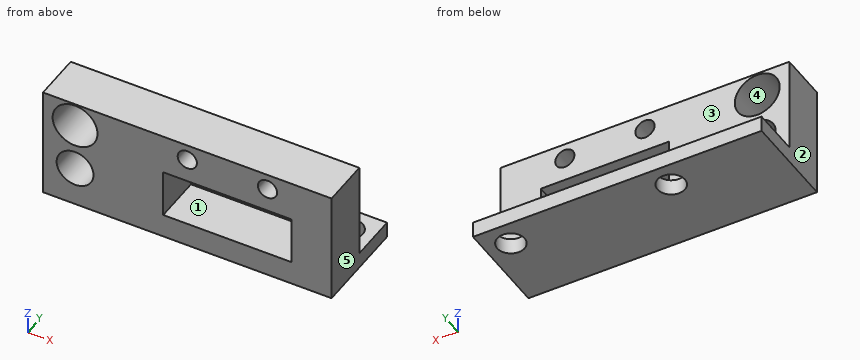
from build123d import *

# Parameters (mm, degrees)
SKETCH1_W           = 45.72
SKETCH1_H           = 17.78
BOSS_EXTRUDE1_DEPTH = 7.62
SKETCH2_W           = 45.72
SKETCH2_H           = 2.54
BOSS_EXTRUDE2_DEPTH = 7.62
SKETCH3_R           = 2.1717
CUT_EXTRUDE1_DEPTH  = 2.54
SKETCH4_R           = 3.556
SKETCH4_R_2         = 2.921
SKETCH4_R_3         = 1.524
SKETCH4_W           = 20.32
SKETCH4_H           = 7.62
CUT_EXTRUDE2_DEPTH  = 7.62


with BuildPart() as part:
    # Sketch1 → Boss-Extrude1 (new body)
    with BuildSketch(Plane(origin=(0, 0, 0), x_dir=(1, 0, 0), z_dir=(0, 1, 0))):
        with Locations((-7.464489796, 4.231173469)):
            Rectangle(SKETCH1_W, SKETCH1_H)
    extrude(amount=BOSS_EXTRUDE1_DEPTH)

    # Sketch2 → Boss-Extrude2 (add)
    with BuildSketch(Plane(origin=(0, 7.62, 0), x_dir=(1, 0, 0), z_dir=(0, 1, 0))):
        with Locations((-7.464489796, 11.851173469)):
            Rectangle(SKETCH2_W, SKETCH2_H)
    extrude(amount=BOSS_EXTRUDE2_DEPTH)

    # Sketch3 → Cut-Extrude1 (cut)
    with BuildSketch(Plane(origin=(0, 0, -13.121173469), x_dir=(-1, 0, 0), z_dir=(0, 0, -1))):
        with Locations((13.814489796, 11.43)):
            Circle(SKETCH3_R)
        with Locations((-11.585510204, 11.43)):
            Circle(SKETCH3_R)
    extrude(amount=-CUT_EXTRUDE1_DEPTH, mode=Mode.SUBTRACT)

    # Sketch4 → Cut-Extrude2 (cut)
    with BuildSketch(Plane(origin=(0, 7.62, 0), x_dir=(1, 0, 0), z_dir=(0, 1, 0))):
        with Locations(Location((-25.244489796, -0.848826531, 0), (0, 0, 270))):
            Circle(SKETCH4_R)
        with Locations(Location((-25.244489796, 6.771173469, 0), (0, 0, 270))):
            Circle(SKETCH4_R_2)
        with Locations(Location((-7.464489796, -2.118826531, 0), (0, 0, 270))):
            Circle(SKETCH4_R_3)
        with Locations(Location((5.235510204, -2.118826531, 0), (0, 0, 270))):
            Circle(SKETCH4_R_3)
        with Locations((-1.114489796, 5.501173469)):
            Rectangle(SKETCH4_W, SKETCH4_H)
    extrude(amount=-CUT_EXTRUDE2_DEPTH, mode=Mode.SUBTRACT)


solid = part.part
Read the model definition and answer for the solid it produces. Units are mm, in the model's axes. Face numbers are marked on the shaded views. A direction names the side the tool comes from. Round coordinates to 2 decimals unless told otherwise and drop trailing zeros. Loops run counter-clockwise (first coordinate to the right, second up) from the corner with the lowest first, then second, coordinate; pieces in that order, holes last.
Q1. Section D-D on x = -24.5 is taken. Write down the section's boundary in (y, z), and give its area (3 significant figures).
Q2. Section A-A on x = 7.5 is taken. Write down the section's boundary in (y, z), and give its area (3 significant figures).
Q3. Determine the mould class of the marked faces 3, 4 and 5 for opening direction X: released by +X, released by -X, zero draft, split by the parting line, or undercut.
Q4. Consider probe 1 along X at (y, z) = (4.5, -9.25); probe 2 along X at (y, z) = (1.75, -7.25); probe 3 along Z at (x, y) = (6, 7.5). Determine where each line is inside the solid, lowest interval first.
Q5. Each of these flat-tipped pins is pushed along its axis until it touches: pin 1 (2.5 mm diameter, centred on x = -7.5, y = 11, fed in from +Z); pin 2 (6 mm diameter, centred on x = -13, z = -0.5, fed in from +Y). Where does it stop, or does it pass through?
Q6. Section B-B on y = 11.43 is taken. Write down the section's boundary in (x, z).
Q7. Section C-C on z = -7.5 is taken. Write down the section's boundary in (x, y).
Q8. Which of the six approach directions +Z, -Z, +X, -X, +Y, -Y give full straight-line access (tool end or side, diameter ignored) to the marked faces 1 and 2?
Output:
1. outline: (0, -13.12) - (15.24, -13.12) - (15.24, -10.58) - (7.62, -10.58) - (7.62, -9.6) - (0, -9.6) - close; (0, -3.95) - (7.62, -3.95) - (7.62, -2.63) - (0, -2.63) - close; (0, 4.33) - (7.62, 4.33) - (7.62, 4.66) - (0, 4.66) - close
1. area: 58.8 mm2
2. outline: (0, -13.12) - (15.24, -13.12) - (15.24, -10.58) - (7.62, -10.58) - (7.62, -9.31) - (0, -9.31) - close; (0, -1.69) - (7.62, -1.69) - (7.62, 4.66) - (0, 4.66) - close
2. area: 96.8 mm2
3. face 3: zero draft
3. face 4: undercut
3. face 5: released by +X
4. probe 1: x = -30.32 to -26.79, -23.7 to -11.27, 9.05 to 15.4
4. probe 2: x = -30.32 to -28.13, -22.36 to -11.27, 9.05 to 15.4
4. probe 3: z = -13.12 to -9.31, -1.69 to 0.8, 3.44 to 4.66
5. pin 1: stops at z = -10.58
5. pin 2: stops at y = 7.62
6. outline: (-30.32, -13.12) - (-15.99, -13.12) - (-15.99, -10.58) - (-30.32, -10.58) - close; (-11.64, -13.12) - (9.41, -13.12) - (9.41, -10.58) - (-11.64, -10.58) - close; (13.76, -13.12) - (15.4, -13.12) - (15.4, -10.58) - (13.76, -10.58) - close
7. outline: (-30.32, 0) - (-28.07, 0) - (-28.07, 7.62) - (-30.32, 7.62) - close; (-22.42, 0) - (-11.27, 0) - (-11.27, 7.62) - (-22.42, 7.62) - close; (9.05, 0) - (15.4, 0) - (15.4, 7.62) - (9.05, 7.62) - close
8. face 1: +Y, -Y
8. face 2: +Z, -Z, -X, +Y, -Y
